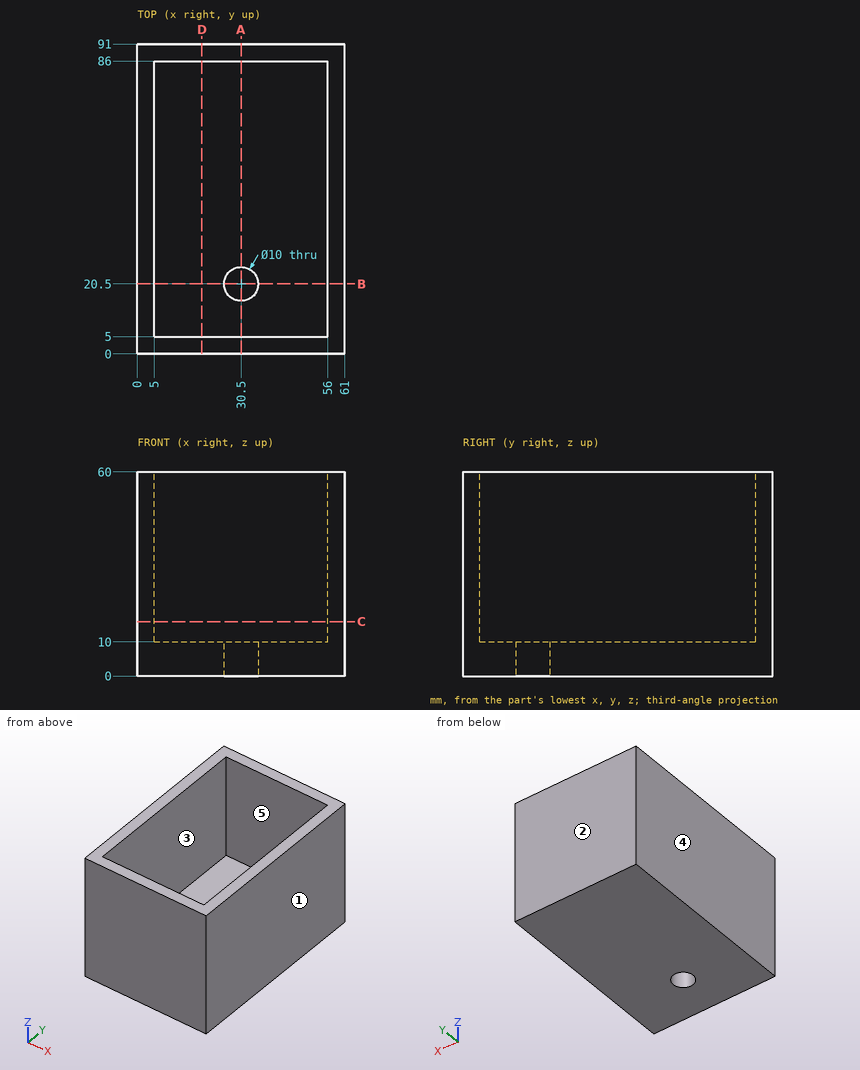
Print and shaded views of the part. All mm, measured from the part's lowest x, y and z. A direction names the side the tool comes from. Coordinates: 2 decimals unless noted, no trailing zeros. Order: outer loops, then holes, each group sorted by start corner. A loop starts at its lowest first (then second) coordinate and runs counter-clockwise, first axis right, second up. Notation, with made-up numbers: M 50.5,-3.75 L 72.5,-3.75 A13 cw 72.5,1.25 Z; hole C 61.5,20 d6. An arc over 180 degrees is marked long. Answer as CSV lines item,"result".
1) Cut at B-B (y = 20.5). List the corners of the cut face in (x, z).
Verdict:
outline,"M 0,0 L 25.5,0 L 25.5,10 L 5,10 L 5,60 L 0,60 Z; M 35.5,0 L 61,0 L 61,60 L 56,60 L 56,10 L 35.5,10 Z"
2) Cut at A-A (x = 30.5). List the corners of the cut face in (y, z).
Verdict:
outline,"M 0,0 L 15.5,0 L 15.5,10 L 5,10 L 5,60 L 0,60 Z; M 25.5,0 L 91,0 L 91,60 L 86,60 L 86,10 L 25.5,10 Z"
3) Flat gauge pins, fed straight in: P1, Ø6, axis at y = 77, z = 52, coming from the -X side; P2, Ø1.5, axis at x = 16, y = 29.5, coming from the +Z side; P3, Ø9, axis at x = 30.5, y = 20.5, coming from the -Z side. Where does each tip first touch, or does it go through?
Verdict:
P1,"x = 0"
P2,"z = 10"
P3,"through"
4) Cut at D-D (x = 19). List the corners of the cut face in (y, z).
Verdict:
outline,"M 0,0 L 91,0 L 91,60 L 86,60 L 86,10 L 5,10 L 5,60 L 0,60 Z"
5) Drill centre lines: L1, parallel to Y at x = 9.5, z = 48; L2, parallel to X at y = 50, z = 20.5; L3, parallel to X at y = 20, z = 2. Where is each one in solid material? Low to high. Write a range as from..to.
Verdict:
L1,"0..5, 86..91"
L2,"0..5, 56..61"
L3,"0..25.53, 35.47..61"
6) Cut at C-C (z = 16). List the corners of the cut face in (x, y), then the cut area to 3 significant figures.
Verdict:
outline,"M 0,0 L 61,0 L 61,91 L 0,91 Z; hole M 5,5 L 56,5 L 56,86 L 5,86 Z"
area,"1,420 mm2"
7) Mould opens along Y. For the marked faces 1, 2 and 3 say: released by +Y, released by -Y, zero draft, split by the parting line, or undercut.
Verdict:
face 1,"zero draft"
face 2,"released by +Y"
face 3,"undercut"
8) 3-axis set-ups, long thin cutter, end or side, ignore diameter. For the marked faces 4 and 5: which of +Z, -Z, +X, -X, +Y, -Y reach the whole face in a straight line?
Verdict:
face 4,"+Z, -Z, -X, +Y, -Y"
face 5,"+Z"
